Build history of the part. All positions in model axes, mm. A direction names the side the tool comes from. Round coordinates to 2 decimals unless told otherwise and drop trailing zeros. Loops run counter-clockwise (first coordinate to the right, second up) from the corner with the lowest first, then second, coordinate; pieces in that order, holes last. Notation, with made-up numbers: M 33.25,54.5 L 72.25,54.5 A20 cw 72.25,67.5 Z; hole C 0,39 d6. An arc over 180 degrees is marked long. One line per item, written item: value.
```python
from build123d import *

# Parameters (mm, degrees)
SKETCH2_W           = 12.7
SKETCH2_H           = 12.7
SKETCH2_H_2         = 0.5
BOSS_EXTRUDE2_DEPTH = 0.5
SKETCH2_4_W         = 12.7
SKETCH2_4_H         = 0.5
BOSS_EXTRUDE3_DEPTH = 15
SKETCH3_W           = 13.7
SKETCH3_H           = 1
BOSS_EXTRUDE4_DEPTH = 7
SKETCH4_W           = 13.7
SKETCH4_H           = 1
BOSS_EXTRUDE6_DEPTH = 7


with BuildPart() as part:
    # Sketch2 → Boss-Extrude2 (new body)
    with BuildSketch(Plane(origin=(0, 0, 0), x_dir=(1, 0, 0), z_dir=(0, 1, 0))):
        with Locations((6.85, 6.85)):
            Rectangle(SKETCH2_W, SKETCH2_H)
        Polygon((13.2, 0.5), (13.2, 0), (13.7, 0), (13.7, 13.7), (13.2, 13.7), (13.2, 13.2), align=None)
        with Locations((6.85, 13.45)):
            Rectangle(SKETCH2_W, SKETCH2_H_2)
        Polygon((0, 0.5), (0, 0), (13.2, 0), (13.2, 0.5), (0.5, 0.5), align=None)
        Polygon((0, 13.7), (0, 0.5), (0.5, 0.5), (0.5, 13.2), (0.5, 13.7), align=None)
    extrude(amount=-BOSS_EXTRUDE2_DEPTH)

    # Sketch2_4 → Boss-Extrude3 (add)
    with BuildSketch(Plane(origin=(0, 0, 0), x_dir=(1, 0, 0), z_dir=(0, 1, 0))):
        Polygon((0, 13.7), (0, 0.5), (0.5, 0.5), (0.5, 13.2), (0.5, 13.7), align=None)
        with Locations((6.85, 13.45)):
            Rectangle(SKETCH2_4_W, SKETCH2_4_H)
        Polygon((13.2, 0.5), (13.2, 0), (13.7, 0), (13.7, 13.7), (13.2, 13.7), (13.2, 13.2), align=None)
        Polygon((0, 0.5), (0, 0), (13.2, 0), (13.2, 0.5), (0.5, 0.5), align=None)
    extrude(amount=BOSS_EXTRUDE3_DEPTH)

    # Sketch3 → Boss-Extrude4 (add)
    with BuildSketch(Plane.XY):
        with Locations((6.85, 0)):
            Rectangle(SKETCH3_W, SKETCH3_H)
    extrude(amount=BOSS_EXTRUDE4_DEPTH)

    # Sketch4 → Boss-Extrude6 (add)
    with BuildSketch(Plane(origin=(0, 0, -13.7), x_dir=(-1, 0, 0), z_dir=(0, 0, -1))):
        with Locations((-6.85, 0)):
            Rectangle(SKETCH4_W, SKETCH4_H)
    extrude(amount=BOSS_EXTRUDE6_DEPTH)


solid = part.part
```
Item 1: Slice it at A-A, the plane y = 11.5. Give the cut face in (x, z), and give its area (3 significant figures).
Check values:
outline: M 0,-13.7 L 13.7,-13.7 L 13.7,0 L 0,0 Z; hole M 0.5,-13.2 L 13.2,-13.2 L 13.2,-0.5 L 0.5,-0.5 Z
area: 26.4 mm2
Item 2: Slice it at C-C, the plane x = 11.75. Give the cut face in (y, z).
Check values:
outline: M -0.5,-20.7 L 0.5,-20.7 L 0.5,-13.7 L 15,-13.7 L 15,-13.2 L 0,-13.2 L 0,-0.5 L 15,-0.5 L 15,0 L 0.5,0 L 0.5,7 L -0.5,7 Z
Item 3: Drop flat-ended pins along their axis: P1, Ø3, axis at x = 1.5, y = 13, coming from the -Z side; P2, Ø2, axis at x = 6, z = 2.5, coming from the +Y side; P3, Ø6.5, axis at x = 8, y = 10.5, coming from the +Z side. Give the stop position or say it passes through.
Check values:
P1: stops at z = -13.7
P2: stops at y = 0.5
P3: stops at z = 0
Item 4: Pull direction Z, two halves, no side cores. Call faces 5 (the face through (0.5, 7, -7)), 6 (the face through (7, 0, 7)), 7 (the face through (7, 0.5, -17)), 8 (the face through (7, 0, -20.7)): pulls with the +Z half, pulls with the -Z half, needs draft (parallel to the pull), parting line crosses it, or undercut.
Check values:
face 5: undercut
face 6: pulls with the +Z half
face 7: needs draft
face 8: pulls with the -Z half
Item 5: Slice it at B-B, the plane z = -9.75. Give the cut face in (x, y).
Check values:
outline: M 0,-0.5 L 13.7,-0.5 L 13.7,15 L 13.2,15 L 13.2,0 L 0.5,0 L 0.5,15 L 0,15 Z
Item 6: Wall check: line 1 along Z through (x, y) = (11.25, 8); line 2 along X through (y, z) = (2, -5.5); line 3 along Y through (x, z) = (3.5, 2). Give the ranges that are in metal, low to high.
Check values:
line 1: z = -13.7 to -13.2, -0.5 to 0
line 2: x = 0 to 0.5, 13.2 to 13.7
line 3: y = -0.5 to 0.5
Item 7: Which spindle directions (+Z, -Z, +X, -X, +Y, -Y) get a long thin tool onto all of the face, cutting with end or side? Do faces 1 (the face through (7, -0.5, -7)), 2 (the face through (7, 0.5, 3)), 3 (the face through (7, 8, -13.7)), 4 (the face through (7, 7, -13.2)). Say none if no direction does.
Check values:
face 1: +Z, -Z, +X, -X, -Y
face 2: +Z, +X, -X, +Y
face 3: -Z, +X, -X, +Y
face 4: +Y
Item 8: Slice it at D-D, the plane z = -15.75. Give the cut face in (x, y), and give its area (3 significant figures).
Check values:
outline: M 0,-0.5 L 13.7,-0.5 L 13.7,0.5 L 0,0.5 Z
area: 13.7 mm2
